Verification items for the finished model (mm, model axes). A direction names the side the tool comes from. Round coordinates to 2 decimals unless told otherwise and drop trailing zeros. Order: outer loops, then holes, each group sorted by start corner. A loop starts at its lowest first (then second) coordinate and runs counter-clockwise, first axis right, second up. Notation, with made-up numbers: M -30.5,-12 L -23.5,-12 A13 cw -23.5,12 Z; hole C 82,-16.5 d11. An arc over 180 degrees is marked long. Return JSON: item names as keys, results as strings. Group by question number.
Autodesk Inventor part; units mm, degrees
ref_plane "Work Plane1" through (29, 0, 0) normal (0, -1, 0) x (1, 0, 0)
ref_plane "YZ Plane" through (0, 0, 0) normal (1, 0, 0) x (0, 1, 0)
ref_plane "XZ Plane" through (0, 0, 0) normal (0, 1, 0) x (-1, 0, 0)
sketch "Sketch1" plane through (0, 0, 0) normal (0, 0, 1) x (1, 0, 0)
  line L0 (-0.8667, 0) -> (15, 0)
  line L1 (15, 0) -> (15, 1.5)
  line L2 (15, 1.5) -> (4.25, 1.5)
  line L3 (4.25, 1.5) -> (3.9432, 1.5)
  line L4 (3.9432, 1.5) -> (0, 1.5)
  line L5 (0, 1.5) -> (0, 2.75)
  line L6 (0, 2.75) -> (-3, 2.75)
  line L7 (-3, 2.75) -> (-3, 1.4434)
  line L8 (-3, 1.4434) -> (-1.7, 1.4434)
  line L9 (-1.7, 1.4434) -> (-0.8667, 0)
  line L10 (-6.6, 0) -> (18.6, 0)
  line L11 (0, -0.55) -> (0, 3.3)
  line L12 (4.25, 1.5) -> (0, 1.5) construction
  dimension "d1" = 10.75
  dimension "d2" = 0.3068
  dimension "d3" = 3
  dimension "d4" = 1.3
  dimension "d5" = 60
  dimension "d6" = 3
  dimension "d7" = 3
  dimension "d8" = 2.8868
  dimension "d9" = 5.5
  dimension "d26" = 15
revolve "Body" add sketch "Sketch1" angle 360 about axis through (-0.8667, 0, 0) along (1, 0, 0)
sketch "Sketch2" plane through (-3, 0, 0) normal (-1, 0, 0) x (0, 0, 1)
  circle A0 centre (0, 0) radius 1.4434
  line L0 (0, -3.85) -> (0, 3.85)
  line L1 (-3.85, 0) -> (3.85, 0)
  line L2 (1.4434, 0) -> (0.7217, -1.25)
  line L3 (0.7217, -1.25) -> (-0.7217, -1.25)
  line L4 (-0.7217, -1.25) -> (-1.4434, 0)
  line L5 (-1.4434, 0) -> (-0.7217, 1.25)
  line L6 (-0.7217, 1.25) -> (0.7217, 1.25)
  line L7 (0.7217, 1.25) -> (1.4434, 0)
  point P0 (0, 0)
extrude "Slot" add sketch "Sketch2" against normal up to next contours L7 A0 | A0 L2 | L6 L0 A0 | A0 L0 L3 | L0 L6 A0 | A0 L3 L0 | L4 A0 | A0 L5
fillet "Fillet1" radius 0.3 1 edges at (-3, -2.75, 0)
thread "Thread"
chamfer "Chamfer1" distance 0.3067 distance2 0.3067 1 edges at (15, -1.5, 0) measured on face at (15, 0.5539, 0.4443)
ref_plane "Work Plane1" through (29, 0, 0) normal (0, -1, 0) x (1, 0, 0)
fillet "Fillet2" radius 0.1 1 edges at (0, -1.5, 0)
equation "\"d1\" = GEL"
equation "\"d3\" = KOH"
equation "\"d4\" = INTI"
equation "\"d6\" = GD"
equation "\"d7\" = BDM"
equation "\"d8\" = 1.1547 * SW"
equation "\"d9\" = KOD"
equation "\"d30\" = R"
equation "\"d17\" = RR"
equation "\"d13\" = GEL"
equation "\"d15\" = -0.5 * SPD + 0.5 * GD"
equation "\"d16\" = GUL"
equation "\"GD\" = NND"
equation "\"NLG\" = 12"
equation "\"GEL\" = 10.75"
equation "\"KOD\" = 5.5"
equation "\"KOH\" = NND"
equation "\"INTI\" = 1.3"
equation "\"GAL\" = 0.61345 * PTC"
equation "\"GUL\" = 0.61345 * PTC"
equation "\"BDM\" = NND"
equation "\"SW\" = 2.5"
equation "\"RR\" = 0.1 * NND"
equation "\"SPD\" = NND - 1.2269 * PTC"
equation "\"R\" = 0.1"
equation "\"PHH\" = 0.13"
equation "\"GD1\" = THREADDIA - 1.2269 * PTC"
equation "\"THREADDIA\" = 3"
equation "\"FAWI\" = 45deg"
equation "\"PTC\" = 0.5"
equation "\"KOH1\" = 2.7"
equation "\"NND\" = 3"
equation "\"TOA\" = 30deg"
equation "\"E0\" = 1.155 * SW"
properties part number "F105" material "Steel, Mild"
1. Draft check along Y on faces 3 (the face through (7.29, -1.5, -0.07)), 4 (the face through (0, 2, 0)), 5 (the face through (-2.3, 0.63, 1.08)). Enter one of: +Y half, -Y half, draft (parallel to the pull), parting line (faces both ways), or undercut.
2. Access from +Z, -Z, +X, -X, +Y, -Y to the whole of each face (thin tool, end or side, straight path). Record for faces 1 (the face through (-2, 1.25, 0)), 2 (the face through (15, 0, 0)).
3. Cross-section at A-A (x = 7.5). Enter the section's corners in (y, z).
4. Thickness scan on line 1 along X through (y, z) = (1.95, -1.45); line 2 along Y through (x, z) = (11, -1.15); line 3 along Y through (x, z) = (10.5, 1.35). Record the ranges inside material, lowest first. Write a range as from..to.
5. Go/stop test with flat-tipped pins: pin 1 (1.5 mm diameter, centred on x = 9, z = -1.5, fed in from -Y); pin 2 (1.5 mm diameter, centred on x = 4, z = 1.5, fed in from +Y); pin 3 (3 mm diameter, centred on x = 11, y = -0.5, fed in from +Z). Record where each tip stops, or that it passes through.
Computed:
{
 "1": {"face 3": "parting line", "face 4": "draft", "face 5": "undercut"},
 "2": {"face 1": "-X", "face 2": "+Z, -Z, +X, +Y, -Y"},
 "3": {"outline": "C 0,0 d3"},
 "4": {"line 1": "x = -3..0", "line 2": "y = -0.96..0.96", "line 3": "y = -0.65..0.65"},
 "5": {"pin 1": "stops at y = -1.3", "pin 2": "stops at y = 1.3", "pin 3": "stops at z = 1.5"}
}
